Work out the finished part from the listing and answer in its coordinate system (mm). Face numbers are marked on the shaded views. Round coordinates to 2 decimals unless told otherwise and drop trailing zeros. Loops run counter-clockwise (first coordinate to the right, second up) from the corner with the lowest first, then second, coordinate; pieces in that order, holes last. Notation, with made-up numbers: (10, 74.25) -> (67, 74.25) arc R20 ccw to (67, 98.25) -> close; hole circle Ø1 at (41, 81.5). An arc over 180 degrees is marked (long way). Use CSV: the item, a comma, the result in double quotes. Start each with the question number.
from build123d import *

# Parameters (mm, degrees)
SKETCH1_R           = 2.5
BOSS_EXTRUDE1_DEPTH = 3
SKETCH2_R           = 3


with BuildPart() as part:
    # Sketch1 → Boss-Extrude1 (new body)
    with BuildSketch(Plane(origin=(0, 0, 0), x_dir=(1, 0, 0), z_dir=(0, 1, 0))):
        with BuildLine():
            Line((15, -17.5), (-15, -17.5))
            ThreePointArc((-15, -17.5), (-18.535533906, -16.035533906), (-20, -12.5))
            Line((-20, -12.5), (-20, 12.5))
            ThreePointArc((-20, 12.5), (-18.535533906, 16.035533906), (-15, 17.5))
            Line((-15, 17.5), (15, 17.5))
            ThreePointArc((15, 17.5), (18.535533906, 16.035533906), (20, 12.5))
            Line((20, 12.5), (20, -12.5))
            ThreePointArc((20, -12.5), (18.535533906, -16.035533906), (15, -17.5))
        make_face()
        with Locations(Location((-12.5, 10, 0), (0, 0, 270))):
            Circle(SKETCH1_R, mode=Mode.SUBTRACT)
        with Locations(Location((12.5, 10, 0), (0, 0, 270))):
            Circle(SKETCH1_R, mode=Mode.SUBTRACT)
        with Locations(Location((-12.5, -10, 0), (0, 0, 270))):
            Circle(SKETCH1_R, mode=Mode.SUBTRACT)
        with Locations(Location((12.5, -10, 0), (0, 0, 270))):
            Circle(SKETCH1_R, mode=Mode.SUBTRACT)
    extrude(amount=BOSS_EXTRUDE1_DEPTH)

    # Sweep1: sweep along a path in Sketch3
    with BuildLine(Plane.XY) as sweep1_path:
        Line((-10, 0), (-10, 14.2))
        ThreePointArc((-10, 14.2), (0, 24.2), (10, 14.2))
        Line((10, 14.2), (10, 0))
    # Sketch2 → Sweep1 (sweep)
    with BuildSketch(Plane(origin=(0, 0, 0), x_dir=(1, 0, 0), z_dir=(0, 1, 0))):
        with Locations((-10, 0)):
            Circle(SKETCH2_R)
    sweep(path=sweep1_path.line)


solid = part.part
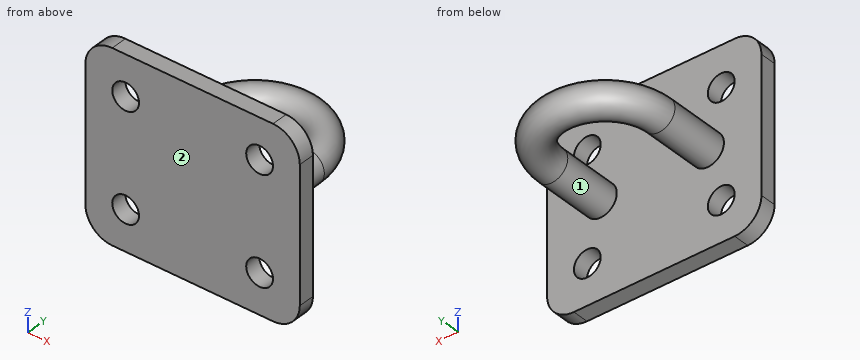
Q1. Section B-B, the plane y = 2 is taken. Write down the section's boundary in (x, z).
Q2. Section C-C, the plane z = 0 is taken. Write down the section's boundary in (x, y), and give its area (3 significant figures).
Q3. Each of these flat-tipped pins is pushed along its axis until it touches: pin 1 (2 mm diameter, centred on x = -2.5, z = -13, fed in from +Y); pin 2 (8 mm diameter, centred on x = 10.5, y = 22, fed in from -Z); pin 3 (12 mm diameter, centred on x = -11.5, z = -3, fed in from +Y). Where does it stop, or does it pass through?
Q4. Section A-A, the plane z = 10 is taken. Write down the section's boundary in (x, y), and give its area (3 significant figures).
Q5. Section D-D, the plane y = 11.5 is taken. Write down the section's boundary in (x, z).
Q6. For a pull along Y with two mould halves and no side action, classify the marked faces 1 and 2 as pulls with the +Y half, pulls with the -Y half, needs draft (parallel to the pull), parting line crosses it, or undercut.
Q7. Straight lines are drawn through the part: line 1 (X direction, y = 2.3, z = -10); line 2 (Y direction, x = -10, z = -4); line 3 (X direction, y = 2.5, z = -11.5). For each, find the intervals that lie inside material, in ascending order. Write a range as from..to.
Report:
1,outline,"(-20, -12.5) arc R5 ccw to (-15, -17.5) -> (15, -17.5) arc R5 ccw to (20, -12.5) -> (20, 12.5) arc R5 ccw to (15, 17.5) -> (-15, 17.5) arc R5 ccw to (-20, 12.5) -> close; hole circle Ø5 at (-12.5, -10); hole circle Ø5 at (-12.5, 10); hole circle Ø5 at (12.5, -10); hole circle Ø5 at (12.5, 10)"
2,outline,"(-20, 0) -> (20, 0) -> (20, 3) -> (13, 3) -> (13, 14.2) arc R13 ccw to (-13, 14.2) -> (-13, 3) -> (-20, 3) -> close; hole (-7, 3) -> (7, 3) -> (7, 14.2) arc R7 ccw to (-7, 14.2) -> close"
2,area,"443 mm²"
3,pin 1,"stops at y = 3"
3,pin 2,"stops at z = -3"
3,pin 3,"stops at y = 25.66"
4,outline,"(-20, 0) -> (-15, 0) -> (-15, 3) -> (-20, 3) -> close; (-10, 0) -> (10, 0) -> (10, 3) -> (-10, 3) -> close; (15, 0) -> (20, 0) -> (20, 3) -> (15, 3) -> close"
4,area,"90.0 mm²"
5,outline,"circle Ø6 at (-10, 0); circle Ø6 at (10, 0)"
6,face 1,"undercut"
6,face 2,"pulls with the -Y half"
7,line 1,"x = -20..-15, -10..10, 15..20"
7,line 2,"y = 0..3"
7,line 3,"x = -20..-14.5, -10.5..10.5, 14.5..20"
